Design review of the part built by this model. Coordinates are the model's own, in mm. Coordinates: 2 decimals unless noted, no trailing zeros. Loops run counter-clockwise (first coordinate to the right, second up) from the corner with the lowest first, then second, coordinate; pieces in that order, holes last. Notation, with made-up numbers: M -17,-12.5 L 2,-12.5 A10 ccw 2,-0.5 Z; hole C -15.75,-2.5 d11. An arc over 180 degrees is marked long. One line per item, written item: value.
```python
from build123d import *

# Parameters (mm, degrees)
SKETCH1_W           = 8.2
SKETCH1_H           = 3.33
BOSS_EXTRUDE1_DEPTH = 0.785
SKETCH2_W           = 8.2
SKETCH2_H           = 2.88
BOSS_EXTRUDE2_DEPTH = 4.15
FILLET1_R           = 1
FILLET2_R           = 0.3
SKETCH3_W           = 2
SKETCH3_H           = 3
BOSS_EXTRUDE3_DEPTH = 0.45


with BuildPart() as part:
    # Sketch1 → Boss-Extrude1 (new body)
    with BuildSketch(Plane.XY):
        with Locations((0, 1.215)):
            Rectangle(SKETCH1_W, SKETCH1_H)
    extrude(amount=BOSS_EXTRUDE1_DEPTH)

    # Sketch2 → Boss-Extrude2 (add)
    with BuildSketch(Plane(origin=(0, 0, 0), x_dir=(-1, 0, 0), z_dir=(0, 0, -1))):
        with Locations((0, 1.44)):
            Rectangle(SKETCH2_W, SKETCH2_H)
    extrude(amount=BOSS_EXTRUDE2_DEPTH)

    # Fillet1
    fillet1_edges = [part.edges().sort_by_distance(p)[0] for p in [
        (-4.1, 2.88, -1.6825),
        (4.1, 2.88, -1.6825),
    ]]
    fillet(fillet1_edges, radius=FILLET1_R)

    # Fillet2
    fillet2_edges = [part.edges().sort_by_distance(p)[0] for p in [
        (4.1, -0.45, 0.3925),
        (-4.1, -0.45, 0.3925),
    ]]
    fillet(fillet2_edges, radius=FILLET2_R)

    # Sketch3 → Boss-Extrude3 (add)
    with BuildSketch(Plane.XZ):
        with Locations((2.5, -1.5)):
            Rectangle(SKETCH3_W, SKETCH3_H)
        with Locations((-2.5, -1.5)):
            Rectangle(SKETCH3_W, SKETCH3_H)
    extrude(amount=BOSS_EXTRUDE3_DEPTH)


solid = part.part
```
(1) We need section D-D on x = 0.5. State the section outline as (y, z) points (3 decimals).
Reply:
outline: M -0.45,0 L 0,0 L 0,-4.15 L 2.88,-4.15 L 2.88,0.785 L -0.45,0.785 Z
(2) Mouldability with a two-part tool opening along X and no side actions: class faces 1 (the flat face through (0, 1, 0.785)), 2 (the flat face through (-4.1, 1, -2)), 3 (the flat face through (0, 0, -3)) as released by +X, released by -X, zero draft, split by the parting line, or undercut.
Reply:
face 1: zero draft
face 2: released by -X
face 3: undercut
(3) Insertion check: pin 1 (1.2 mm diameter, centred on x = -1, z = -1.5, fed in from -Y). The pin has a flat end and moves straight along its axis. Give the tip position at first contact, or say it passes through.
Reply:
pin 1: stops at y = -0.45
(4) We need section A-A on z = -1.45. State the section outline as (x, y) points, then the cut area to 3 significant figures.
Reply:
outline: M -4.1,0 L -3.5,0 L -3.5,-0.45 L -1.5,-0.45 L -1.5,0 L 1.5,0 L 1.5,-0.45 L 3.5,-0.45 L 3.5,0 L 4.1,0 L 4.1,1.88 A1 ccw 3.1,2.88 L -3.1,2.88 A1 ccw -4.1,1.88 Z
area: 25.0 mm2
(5) We need section C-C on y = 2.55. State the section outline as (x, z) points (3 decimals), then the cut area to 3 significant figures.
Reply:
outline: M -3.842,-4.15 L 3.842,-4.15 L 3.842,0.785 L -3.842,0.785 Z
area: 37.9 mm2
(6) To check wall thickness, follow line 1 along X through (y, z) = (-0.25, -1.95); line 2 along Z through (x, y) = (0.25, -0.25) (3 decimals); line 3 along Y through (x, z) = (-2.5, -3.05). State the ranges of each line that lie inside material, in increasing order. Write a range as [from, to].
Reply:
line 1: x = [-3.5, -1.5], [1.5, 3.5]
line 2: z = [0, 0.785]
line 3: y = [0, 2.88]
(7) We need section B-B on x = -2.5. State the section outline as (y, z) points (3 decimals).
Reply:
outline: M -0.45,-3 L 0,-3 L 0,-4.15 L 2.88,-4.15 L 2.88,0.785 L -0.45,0.785 Z
